Geometry: see drawing. Coordinates: mm, zero at the bounding-box minimum. A direction names the side the tool comes from. Coordinates: 2 decimals unless noted, no trailing zeros. Order: outer loops, then holes, each group sorted by start corner. A loop starts at its lowest first (then second) coordinate and runs counter-clockwise, first axis right, second up.
Item 1: Mould query, pull axis X, two halves, no side actions, for the marked faces 4, 5, 6 and 7. Classes: released by +X, released by -X, zero draft, split by the parting line, or undercut.
Item 2: Section A-A on x = 5. Return the cut outline in (y, z) (1 decimal), then the cut area to 3 significant figures.
Item 3: Section B-B on z = 6. Return the cut outline in (x, y), then the cut area to 3 significant figures.
Item 4: Ray query, line 1 (Z direction, x = 7.5, y = 23.5); line 2 (Y direction, x = 3.75, z = 9.5) (1 decimal); line 3 (Y direction, x = 4.25, z = 6.5) (1 decimal). Return the intervals inside material, ascending.
Item 5: Reachability of the marked faces 1, 2 and 3 from +Z, -Z, +X, -X, +Y, -Y: full face, straight path, thin tool, end or side. Return the list, or none.
Item 6: Section D-D on x = 9.25. Return the cut outline in (y, z).
Item 7: Section C-C on y = 10.5. Return the cut outline in (x, z).
Item 8: Contact query for flat-ended pins moving along their axis: P1, Ø1.5, axis at x = 6.5, z = 6, coming from the +Y side; P2, Ø2, axis at x = 1.5, z = 6, coming from the -Y side; P3, Ø1.5, axis at x = 6, z = 3, coming from the -Y side. Output: stop coordinate, or through.
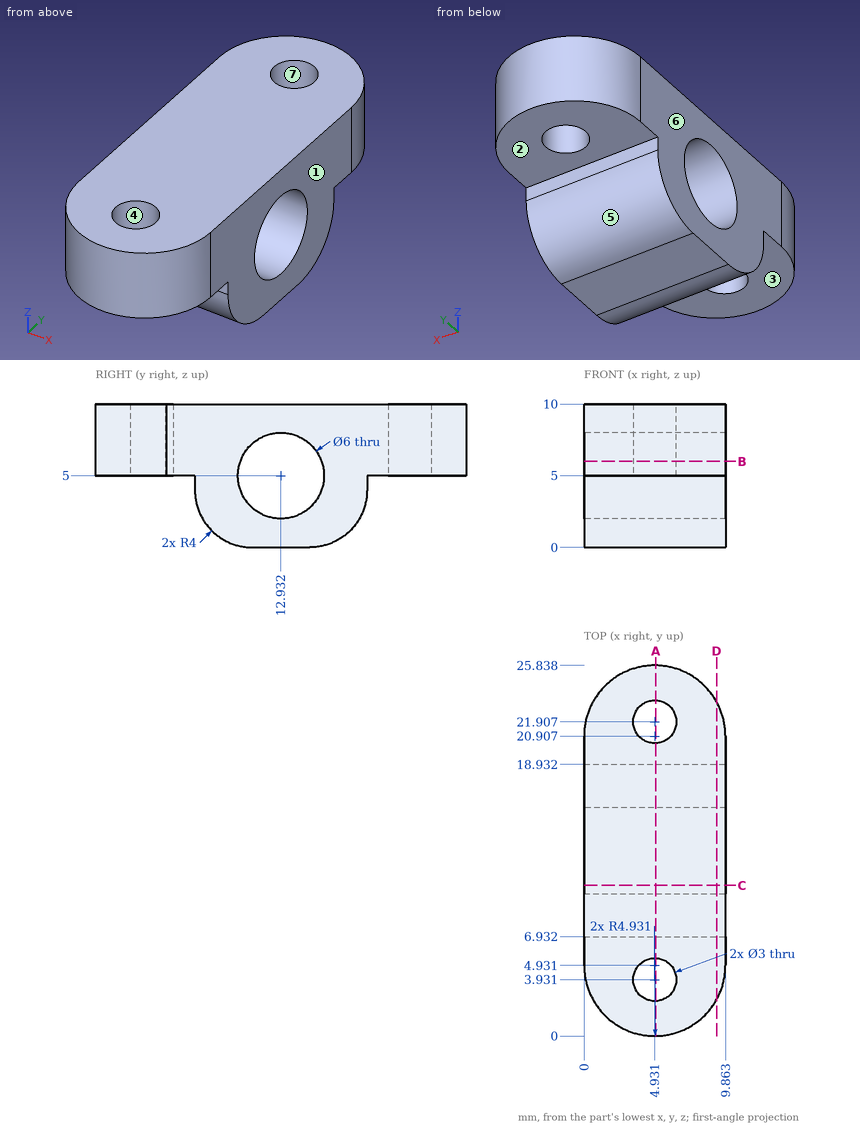
Answer list:
1. face 4: undercut
1. face 5: zero draft
1. face 6: released by -X
1. face 7: undercut
2. outline: (0, 5) - (2.4, 5) - (2.4, 10) - (0, 10) - close; (5.4, 5) - (6.9, 5) - (6.9, 4) arc R4 ccw to (10.9, 0) - (14.9, 0) arc R4 ccw to (18.9, 4) - (18.9, 5) - (20.4, 5) - (20.4, 10) - (5.4, 10) - close; (23.4, 5) - (25.8, 5) - (25.8, 10) - (23.4, 10) - close; hole circle Ø6 at (12.9, 5)
2. area: 124 mm2
3. outline: (0, 4.91) arc R4.93 ccw to (9.86, 4.96) - (9.86, 10.1) - (0, 10.1) - close; (0, 15.76) - (9.86, 15.76) - (9.86, 20.91) arc R4.93 ccw to (0, 20.91) - close; hole circle Ø3 at (4.93, 3.93); hole circle Ø3 at (4.93, 21.91)
3. area: 164 mm2
4. line 1: z = 5 to 10
4. line 2: y = 0.1 to 3, 4.9 to 21, 22.8 to 25.7
4. line 3: y = 0 to 2.6, 5.3 to 10.3, 15.5 to 20.6, 23.2 to 25.8
5. face 1: +Z, -Z, +X, +Y, -Y
5. face 2: -Z, +X, -X, +Y
5. face 3: -Z, +X, -X, -Y
6. outline: (2.55, 5) - (6.93, 5) - (6.93, 4) arc R4 ccw to (10.93, 0) - (14.93, 0) arc R4 ccw to (18.93, 4) - (18.93, 5) - (23.29, 5) - (23.29, 10) - (2.55, 10) - close; hole circle Ø6 at (12.93, 5)
7. outline: (0, 0.02) - (9.86, 0.02) - (9.86, 3.24) - (0, 3.24) - close; (0, 6.76) - (9.86, 6.76) - (9.86, 10) - (0, 10) - close
8. P1: stops at y = 25.77
8. P2: stops at y = 0.64
8. P3: stops at y = 6.94
